Could you check a few things on this model? Use its own coordinates, in mm. Face numbers are marked on the shaded views. A direction names the side the tool comes from. Round coordinates to 2 decimals unless told otherwise and drop trailing zeros. Loops run counter-clockwise (first coordinate to the right, second up) from the corner with the lowest first, then second, coordinate; pieces in that order, holes last. Notation, with made-up numbers: M 83.25,41 L 125.25,41 A21 ccw 125.25,49 Z; hole C 32.25,42.5 d6. An arc over 180 degrees is marked long. Answer in a Markdown table with one row per item.
```python
from build123d import *

# Parameters (mm, degrees)
SKETCH1_R           = 7.5
BOSS_EXTRUDE1_DEPTH = 1.016


with BuildPart() as part:
    # Sketch1 → Boss-Extrude1 (new body)
    with BuildSketch(Plane(origin=(0, 0, 0), x_dir=(1, 0, 0), z_dir=(0, 1, 0))):
        with Locations(Location((0, 0, 0), (0, 0, 270))):
            Circle(SKETCH1_R)
        with BuildLine():
            Line((-0.889, 5.311351523), (-0.889, 4.508))
            ThreePointArc((-0.889, 4.508), (-0.740210245, 4.148789755), (-0.381, 4))
            Line((-0.381, 4), (0.381, 4))
            ThreePointArc((0.381, 4), (0.740210245, 4.148789755), (0.889, 4.508))
            Line((0.889, 4.508), (0.889, 5.311351523))
            ThreePointArc((0.889, 5.311351523), (1.08682242, 5.713662185), (1.526219956, 5.802641868))
            ThreePointArc((1.526219956, 5.802641868), (2.296100594, 5.543277195), (3.023886933, 5.182287894))
            ThreePointArc((3.023886933, 5.182287894), (3.271669773, 4.80866878), (3.127074751, 4.384310608))
            Line((3.127074751, 4.384310608), (2.559019441, 3.816255298))
            ThreePointArc((2.559019441, 3.816255298), (2.410229686, 3.457045053), (2.559019441, 3.097834808))
            Line((2.559019441, 3.097834808), (3.097834808, 2.559019441))
            ThreePointArc((3.097834808, 2.559019441), (3.457045053, 2.410229686), (3.816255298, 2.559019441))
            Line((3.816255298, 2.559019441), (4.384310608, 3.127074751))
            ThreePointArc((4.384310608, 3.127074751), (4.80866878, 3.271669773), (5.182287894, 3.023886933))
            ThreePointArc((5.182287894, 3.023886933), (5.543277195, 2.296100594), (5.802641868, 1.526219956))
            ThreePointArc((5.802641868, 1.526219956), (5.713662185, 1.08682242), (5.311351523, 0.889))
            Line((5.311351523, 0.889), (4.508, 0.889))
            ThreePointArc((4.508, 0.889), (4.148789755, 0.740210245), (4, 0.381))
            Line((4, 0.381), (4, -0.381))
            ThreePointArc((4, -0.381), (4.148789755, -0.740210245), (4.508, -0.889))
            Line((4.508, -0.889), (5.311351523, -0.889))
            ThreePointArc((5.311351523, -0.889), (5.713662185, -1.08682242), (5.802641868, -1.526219956))
            ThreePointArc((5.802641868, -1.526219956), (5.543277195, -2.296100594), (5.182287894, -3.023886933))
            ThreePointArc((5.182287894, -3.023886933), (4.80866878, -3.271669773), (4.384310608, -3.127074751))
            Line((4.384310608, -3.127074751), (3.816255298, -2.559019441))
            ThreePointArc((3.816255298, -2.559019441), (3.457045053, -2.410229686), (3.097834808, -2.559019441))
            Line((3.097834808, -2.559019441), (2.559019441, -3.097834808))
            ThreePointArc((2.559019441, -3.097834808), (2.410229686, -3.457045053), (2.559019441, -3.816255298))
            Line((2.559019441, -3.816255298), (3.127074751, -4.384310608))
            ThreePointArc((3.127074751, -4.384310608), (3.271669773, -4.80866878), (3.023886933, -5.182287894))
            ThreePointArc((3.023886933, -5.182287894), (2.296100594, -5.543277195), (1.526219956, -5.802641868))
            ThreePointArc((1.526219956, -5.802641868), (1.08682242, -5.713662185), (0.889, -5.311351523))
            Line((0.889, -5.311351523), (0.889, -4.508))
            ThreePointArc((0.889, -4.508), (0.740210245, -4.148789755), (0.381, -4))
            Line((0.381, -4), (-0.381, -4))
            ThreePointArc((-0.381, -4), (-0.740210245, -4.148789755), (-0.889, -4.508))
            Line((-0.889, -4.508), (-0.889, -5.311351523))
            ThreePointArc((-0.889, -5.311351523), (-1.08682242, -5.713662185), (-1.526219956, -5.802641868))
            ThreePointArc((-1.526219956, -5.802641868), (-2.296100594, -5.543277195), (-3.023886933, -5.182287894))
            ThreePointArc((-3.023886933, -5.182287894), (-3.271669773, -4.80866878), (-3.127074751, -4.384310608))
            Line((-3.127074751, -4.384310608), (-2.559019441, -3.816255298))
            ThreePointArc((-2.559019441, -3.816255298), (-2.410229686, -3.457045053), (-2.559019441, -3.097834808))
            Line((-2.559019441, -3.097834808), (-3.097834808, -2.559019441))
            ThreePointArc((-3.097834808, -2.559019441), (-3.457045053, -2.410229686), (-3.816255298, -2.559019441))
            Line((-3.816255298, -2.559019441), (-4.384310608, -3.127074751))
            ThreePointArc((-4.384310608, -3.127074751), (-4.80866878, -3.271669773), (-5.182287894, -3.023886933))
            ThreePointArc((-5.182287894, -3.023886933), (-5.543277195, -2.296100594), (-5.802641868, -1.526219956))
            ThreePointArc((-5.802641868, -1.526219956), (-5.713662185, -1.08682242), (-5.311351523, -0.889))
            Line((-5.311351523, -0.889), (-4.508, -0.889))
            ThreePointArc((-4.508, -0.889), (-4.148789755, -0.740210245), (-4, -0.381))
            Line((-4, -0.381), (-4, 0.381))
            ThreePointArc((-4, 0.381), (-4.148789755, 0.740210245), (-4.508, 0.889))
            Line((-4.508, 0.889), (-5.311351523, 0.889))
            ThreePointArc((-5.311351523, 0.889), (-5.713662185, 1.08682242), (-5.802641868, 1.526219956))
            ThreePointArc((-5.802641868, 1.526219956), (-5.543277195, 2.296100594), (-5.182287894, 3.023886933))
            ThreePointArc((-5.182287894, 3.023886933), (-4.80866878, 3.271669773), (-4.384310608, 3.127074751))
            Line((-4.384310608, 3.127074751), (-3.816255298, 2.559019441))
            ThreePointArc((-3.816255298, 2.559019441), (-3.457045053, 2.410229686), (-3.097834808, 2.559019441))
            Line((-3.097834808, 2.559019441), (-2.559019441, 3.097834808))
            ThreePointArc((-2.559019441, 3.097834808), (-2.410229686, 3.457045053), (-2.559019441, 3.816255298))
            Line((-2.559019441, 3.816255298), (-3.127074751, 4.384310608))
            ThreePointArc((-3.127074751, 4.384310608), (-3.271669773, 4.80866878), (-3.023886933, 5.182287894))
            ThreePointArc((-3.023886933, 5.182287894), (-2.296100594, 5.543277195), (-1.526219956, 5.802641868))
            ThreePointArc((-1.526219956, 5.802641868), (-1.08682242, 5.713662185), (-0.889, 5.311351523))
        make_face(mode=Mode.SUBTRACT)
    extrude(amount=BOSS_EXTRUDE1_DEPTH)


solid = part.part
```
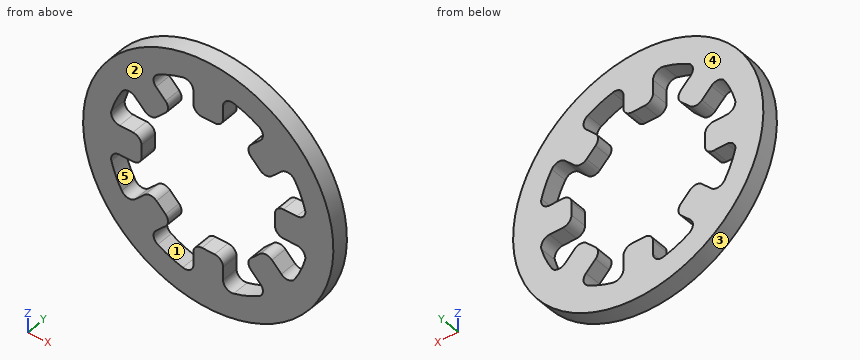
1) I want a section at D-D, the plane z = 6.5. Please give me the cut outline in (x, y).
Computed:
| item | result |
|---|---|
| outline | M -3.74,0 L 3.74,0 L 3.74,1.02 L -3.74,1.02 Z |
2) I need wall thicknesses on line 1 (Z direction, x = 2.5, y = 0.95); line 2 (Z direction, x = 5, y = 0.75); line 3 (X direction, y = 0.2, z = -3). Which ranges of each line are inside material? Lowest first, please.
Computed:
| item | result |
|---|---|
| line 1 | z = -7.07 to -5.45, -3.75 to -3.17, 3.17 to 3.75, 5.45 to 7.07 |
| line 2 | z = -5.59 to -3.21, -0.89 to 0.89, 3.21 to 5.59 |
| line 3 | x = -6.87 to -5.2, -4.26 to -2.66, 2.66 to 4.26, 5.2 to 6.87 |
3) Will these pins go through, and if not, where does the flat tip stop? P1, Ø0.6, axis at y = 0.5, z = 5, coming from the +X side; P2, Ø0.6, axis at x = 5, y = 0.5, coming from the -Z side.
Computed:
| item | result |
|---|---|
| P1 | stops at x = 5.84 |
| P2 | stops at z = -5.84 |
4) I want a section at A-A, the plane z = 0. Please give me the cut outline in (x, y), plus the area to 3 significant figures.
Computed:
| item | result |
|---|---|
| outline | M -7.5,0 L -4,0 L -4,1.02 L -7.5,1.02 Z; M 4,0 L 7.5,0 L 7.5,1.02 L 4,1.02 Z |
| area | 7.11 mm² |
5) Which directions (+Z, -Z, +X, -X, +Y, -Y) give clear straight access to the entire face, cutting with the end or side of a thin tool? Please do the marked faces 1 and 2.
Computed:
| item | result |
|---|---|
| face 1 | +Y, -Y |
| face 2 | +Z, -Z, +X, -X, -Y |
6) I want a section at C-C, the plane z = -6. Please give me the cut outline in (x, y).
Computed:
| item | result |
|---|---|
| outline | M -4.5,0 L 4.5,0 L 4.5,1.02 L -4.5,1.02 Z |
7) I want a section at B-B, the plane x = 0. Please give me the cut outline in (y, z).
Computed:
| item | result |
|---|---|
| outline | M 0,-7.5 L 1.02,-7.5 L 1.02,-4 L 0,-4 Z; M 0,4 L 1.02,4 L 1.02,7.5 L 0,7.5 Z |
8) If we mould it in two halves opening along Z, with no side actions, what happens to the marked faces 3, 4 and 5? For each: released by +Z, released by -Z, zero draft, split by the parting line, or undercut.
Computed:
| item | result |
|---|---|
| face 3 | split by the parting line |
| face 4 | zero draft |
| face 5 | undercut |
